Geometry check sheet. Reference: the model listing, model coordinates, mm. Face numbers are marked on the shaded views. Coordinates: 2 decimals unless noted, no trailing zeros. Write each loop counter-clockwise with the first axis right and the second up, starting at its lowest first coordinate (ties: lowest second). Pieces come first, ordered by that corner, then holes. Notation, with made-up numbers: M 42.25,62.25 L 71.25,62.25 A19 cw 71.25,78.25 Z; hole C 53.25,52 d9. An arc over 180 degrees is marked long. Answer as a JSON object with one key per item and string values. Group by question number.
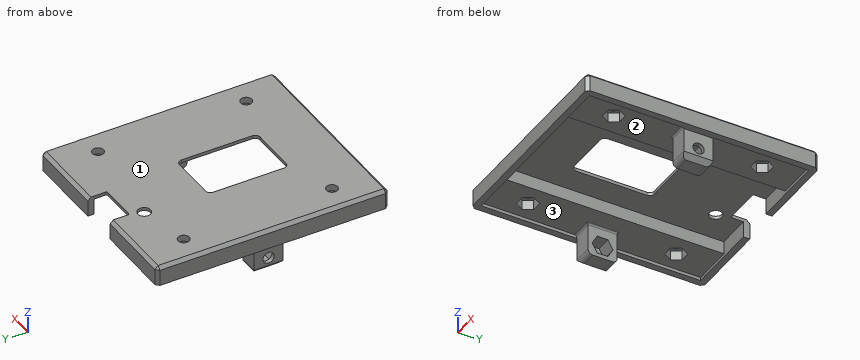
```python
from build123d import *

# Parameters (mm, degrees)
CYLINDER021_R            = 2
CYLINDER021_DEPTH        = 15
BOX014_W                 = 4
BOX014_H                 = 9
BOX014_DEPTH             = 3
PRISM010_DEPTH           = 10
PRISM010_ROLL_ANGLE      = -90.000052
PRISM010_PITCH_ANGLE     = -59.999967
PRISM010_PLACEMENT_ANGLE = 90.000052
CYLINDER019_R            = 1.75
CYLINDER019_DEPTH        = 68
CYLINDER019_PITCH_ANGLE  = 90
BOX013_W                 = 6
BOX013_H                 = 9
BOX013_DEPTH             = 11
CHAMFER008_SIZE          = 1.5
FILLET009_R              = 1.5
BOX012_W                 = 12
BOX012_H                 = 16
BOX012_DEPTH             = 10
PAD021_DEPTH             = 35
CYLINDER005_R            = 1.75
CYLINDER005_DEPTH        = 50
CYLINDER007_R            = 1.75
CYLINDER007_DEPTH        = 50
CYLINDER006_R            = 1.75
CYLINDER006_DEPTH        = 50
CYLINDER004_R            = 1.75
CYLINDER004_DEPTH        = 50
PRISM004_DEPTH           = 10
PRISM005_DEPTH           = 10
PRISM006_DEPTH           = 10
PRISM007_DEPTH           = 10
SKETCH001_W              = 58
SKETCH001_H              = 68
PAD001_DEPTH             = 2
SKETCH002_W              = 33
SKETCH002_H              = 68
PAD002_DEPTH             = 6
BOX009_W                 = 62
BOX009_H                 = 72
BOX009_DEPTH             = 6
CHAMFER001_SIZE          = 1
FILLET010_R              = 0.5


with BuildPart() as cilindro017:
    # Cylinder021 → Cylinder021 (new body)
    with BuildSketch(Plane(origin=(-7, 26, 17), x_dir=(1, 0, 0), z_dir=(0, 0, 1))):
        Circle(CYLINDER021_R)
    extrude(amount=CYLINDER021_DEPTH)


with BuildPart() as cubo014:
    # Box014 → Box014 (new body)
    with BuildSketch(Plane(origin=(-29.75, -4.5, 23), x_dir=(1, 0, 0), z_dir=(0, 0, 1))):
        with Locations((2, 4.5)):
            Rectangle(BOX014_W, BOX014_H)
    extrude(amount=BOX014_DEPTH)


with BuildPart() as prisma010:
    # Prism010 → Prism010 (new body)
    with BuildSketch(Plane.XY):
        Polygon((3.25, 0), (1.625, 2.814583), (-1.625, 2.814583), (-3.25, 0), (-1.625, -2.814583), (1.625, -2.814583), align=None)
    extrude(amount=PRISM010_DEPTH)


with BuildPart() as prisma010_1:
    # Prism010 roll: moved
    add(prisma010.part.rotate(Axis((0, 0, 0), (1, 0, 0)), PRISM010_ROLL_ANGLE))


with BuildPart() as prisma010_2:
    # Prism010 pitch: moved
    add(prisma010_1.part.rotate(Axis((0, 0, 0), (0, 1, 0)), PRISM010_PITCH_ANGLE))


with BuildPart() as prisma010_3:
    # Prism010 placement: moved
    add(prisma010_2.part.moved(Location((-17.5, 0, 18))).rotate(Axis((-17.5, 0, 18), (0, 0, 1)), PRISM010_PLACEMENT_ANGLE))


with BuildPart() as cilindro016:
    # Cylinder019 → Cylinder019 (new body)
    with BuildSketch(Plane.XY):
        Circle(CYLINDER019_R)
    extrude(amount=CYLINDER019_DEPTH)


with BuildPart() as cilindro016_1:
    # Cylinder019 pitch: moved
    add(cilindro016.part.rotate(Axis((0, 0, 0), (0, 1, 0)), CYLINDER019_PITCH_ANGLE))


with BuildPart() as cilindro016_2:
    # Cylinder019 placement: moved
    add(cilindro016_1.part.moved(Location((-34, 0, 18))))


with BuildPart() as fusion016:
    # Box013 → Box013 (new body)
    with BuildSketch(Plane(origin=(-28.75, -4.5, 14), x_dir=(1, 0, 0), z_dir=(0, 0, 1))):
        with Locations((3, 4.5)):
            Rectangle(BOX013_W, BOX013_H)
    extrude(amount=BOX013_DEPTH)

    # Cut028: cut Cilindro016
    add(cilindro016_2.part, mode=Mode.SUBTRACT)

    # Chamfer008
    chamfer008_edges = [fusion016.edges().sort_by_distance(p)[0] for p in [
        (-28.75, 0, 14),
    ]]
    chamfer(chamfer008_edges, length=CHAMFER008_SIZE)

    # Fillet009
    fillet009_edges = [fusion016.edges().sort_by_distance(p)[0] for p in [
        (-25, -4.5, 14),
        (-25, 4.5, 14),
    ]]
    fillet(fillet009_edges, radius=FILLET009_R)

    # Cut029: cut Prisma010
    add(prisma010_3.part, mode=Mode.SUBTRACT)

    # Fusion016: union Cubo014
    add(cubo014.part)


with BuildPart() as part_mirroring032:
    # Part__Mirroring032: instance of Fusion016
    add(fusion016.part.mirror(Plane(origin=(0, 0, 0), x_dir=(0, -1, 0), z_dir=(1, 0, 0))))


with BuildPart() as fusion017:
    # Fusion017 base: copy of Fusion016
    add(fusion016.part)

    # Fusion017: union Part__Mirroring032
    add(part_mirroring032.part)


with BuildPart() as cubo012:
    # Box012 → Box012 (new body)
    with BuildSketch(Plane(origin=(-6, 30, 22), x_dir=(1, 0, 0), z_dir=(0, 0, 1))):
        with Locations((6, 8)):
            Rectangle(BOX012_W, BOX012_H)
    extrude(amount=BOX012_DEPTH)


with BuildPart() as pad021:
    # Sketch018 → Pad021 (new body)
    with BuildSketch(Plane.XY.offset(40)):
        with BuildLine():
            Line((-7, 7), (7, 7))
            ThreePointArc((8.5, 5.5), (8.06066, 6.56066), (7, 7))
            Line((8.5, 5.5), (8.5, -16.5))
            ThreePointArc((7, -18), (8.06066, -17.56066), (8.5, -16.5))
            Line((7, -18), (-7, -18))
            ThreePointArc((-8.5, -16.5), (-8.06066, -17.56066), (-7, -18))
            Line((-8.5, -16.5), (-8.5, 5.5))
            ThreePointArc((-7, 7), (-8.06066, 6.56066), (-8.5, 5.5))
        make_face()
    extrude(amount=-PAD021_DEPTH)


with BuildPart() as cilindro005:
    # Cylinder005 → Cylinder005 (new body)
    with BuildSketch(Plane(origin=(23, 23, -15), x_dir=(1, 0, 0), z_dir=(0, 0, 1))):
        Circle(CYLINDER005_R)
    extrude(amount=CYLINDER005_DEPTH)


with BuildPart() as cilindro007:
    # Cylinder007 → Cylinder007 (new body)
    with BuildSketch(Plane(origin=(23, -23, -15), x_dir=(1, 0, 0), z_dir=(0, 0, 1))):
        Circle(CYLINDER007_R)
    extrude(amount=CYLINDER007_DEPTH)


with BuildPart() as cilindro006:
    # Cylinder006 → Cylinder006 (new body)
    with BuildSketch(Plane(origin=(-23, -23, -15), x_dir=(1, 0, 0), z_dir=(0, 0, 1))):
        Circle(CYLINDER006_R)
    extrude(amount=CYLINDER006_DEPTH)


with BuildPart() as fusion002:
    # Cylinder004 → Cylinder004 (new body)
    with BuildSketch(Plane(origin=(-23, 23, -15), x_dir=(1, 0, 0), z_dir=(0, 0, 1))):
        Circle(CYLINDER004_R)
    extrude(amount=CYLINDER004_DEPTH)

    # Fusion002: union Cilindro005, Cilindro007, Cilindro006
    add(cilindro005.part)
    add(cilindro007.part)
    add(cilindro006.part)


with BuildPart() as prisma004:
    # Prism004 → Prism004 (new body)
    with BuildSketch(Plane(origin=(-23, 23, 0), x_dir=(1, 0, 0), z_dir=(0, 0, 1))):
        Polygon((3.1, 0), (1.55, 2.684679), (-1.55, 2.684679), (-3.1, 0), (-1.55, -2.684679), (1.55, -2.684679), align=None)
    extrude(amount=PRISM004_DEPTH)


with BuildPart() as prisma005:
    # Prism005 → Prism005 (new body)
    with BuildSketch(Plane(origin=(23, 23, 0), x_dir=(1, 0, 0), z_dir=(0, 0, 1))):
        Polygon((3.1, 0), (1.55, 2.684679), (-1.55, 2.684679), (-3.1, 0), (-1.55, -2.684679), (1.55, -2.684679), align=None)
    extrude(amount=PRISM005_DEPTH)


with BuildPart() as prisma006:
    # Prism006 → Prism006 (new body)
    with BuildSketch(Plane(origin=(-23, -23, 0), x_dir=(1, 0, 0), z_dir=(0, 0, 1))):
        Polygon((3.1, 0), (1.55, 2.684679), (-1.55, 2.684679), (-3.1, 0), (-1.55, -2.684679), (1.55, -2.684679), align=None)
    extrude(amount=PRISM006_DEPTH)


with BuildPart() as fusion004:
    # Prism007 → Prism007 (new body)
    with BuildSketch(Plane(origin=(23, -23, 0), x_dir=(1, 0, 0), z_dir=(0, 0, 1))):
        Polygon((3.1, 0), (1.55, 2.684679), (-1.55, 2.684679), (-3.1, 0), (-1.55, -2.684679), (1.55, -2.684679), align=None)
    extrude(amount=PRISM007_DEPTH)

    # Fusion004: union Prisma004, Prisma005, Prisma006
    add(prisma004.part)
    add(prisma005.part)
    add(prisma006.part)


with BuildPart() as fusion004_1:
    # Fusion004 placement: moved
    add(fusion004.part.moved(Location((0, 0, 17))))


with BuildPart() as pad001:
    # Sketch001 → Pad001 (new body)
    with BuildSketch(Plane(origin=(0, 0, 23), x_dir=(1, 0, 0), z_dir=(0, 0, -1))):
        Rectangle(SKETCH001_W, SKETCH001_H)
    extrude(amount=-PAD001_DEPTH)


with BuildPart() as fusion003:
    # Sketch002 → Pad002 (new body)
    with BuildSketch(Plane(origin=(0, 0, 23), x_dir=(1, 0, 0), z_dir=(0, 0, -1))):
        Rectangle(SKETCH002_W, SKETCH002_H)
    extrude(amount=-PAD002_DEPTH)

    # Fusion003: union Pad001
    add(pad001.part)


with BuildPart() as fusion003_1:
    # Fusion003 placement: moved
    add(fusion003.part.moved(Location((0, 0, -1))))


with BuildPart() as obj1:
    # Box009 → Box009 (new body)
    with BuildSketch(Plane(origin=(-31, -36, 23), x_dir=(1, 0, 0), z_dir=(0, 0, 1))):
        with Locations((31, 36)):
            Rectangle(BOX009_W, BOX009_H)
    extrude(amount=BOX009_DEPTH)

    # Chamfer001
    chamfer001_edges = [obj1.edges().sort_by_distance(p)[0] for p in [
        (-31, -36, 26),
        (-31, 0, 29),
        (-31, 36, 26),
        (31, -36, 26),
        (31, 0, 29),
        (31, 36, 26),
        (0, -36, 29),
        (0, 36, 29),
    ]]
    chamfer(chamfer001_edges, length=CHAMFER001_SIZE)

    # Cut004: cut Fusion003
    add(fusion003_1.part, mode=Mode.SUBTRACT)

    # Cut005: cut Fusion004
    add(fusion004_1.part, mode=Mode.SUBTRACT)

    # Cut006: cut Fusion002
    add(fusion002.part, mode=Mode.SUBTRACT)

    # Cut023: cut Pad021
    add(pad021.part, mode=Mode.SUBTRACT)

    # Cut027: cut Cubo012
    add(cubo012.part, mode=Mode.SUBTRACT)

    # Fusion018: union Fusion017
    add(fusion017.part)

    # Fillet010
    fillet010_edges = [obj1.edges().sort_by_distance(p)[0] for p in [
        (-6, 30, 28.5),
        (6, 30, 28.5),
        (-24.25, 4.5, 24),
        (-22.75, 0, 24),
        (-24.25, -4.5, 24),
        (28.875, -4.5, 24),
        (24.25, -4.5, 24),
        (22.75, 0, 24),
        (24.25, 4.5, 24),
    ]]
    fillet(fillet010_edges, radius=FILLET010_R)

    # Cut032: cut Cilindro017
    add(cilindro017.part, mode=Mode.SUBTRACT)


solid = obj1.part
```
1) Section check A-A (x = -18.5). Record the cut outline in (y, z).
2) Section check B-B (y = 10.5). Record the cut outline in (x, z), then the cut area to 3 significant figures.
3) Section check C-C (y = 0). State how many separate pieces and enclosed holes the cut face has, then the cut area to 3 significant figures.
4) Go/stop test with flat-tipped pins: pin 1 Ø12 at (x, y) = (7.5, 1.5) entering from -Z; pin 2 Ø0.5 at (x, z) = (0.5, 28.5) entering from +Y; pin 3 Ø5 at (x, z) = (26.5, 17.5) entering from +Y. Record where each tip stops, or that it passes through.
5) Draft check along X on the marked faces 1, 2 and 3. Enter one of: +X half, -X half, draft (parallel to the pull), parting line (faces both ways), or undercut.
6) Material ranges on probe 1 along X at (y, z) = (23, 27.6); probe 2 along Y at (x, z) = (-7, 26.25); probe 3 along X at (y, z) = (23, 28.1), recorded low to high. Write a range as [from, to].
Entries:
{
 "1": {"outline": "M -36,23 L -34,23 L -34,24 L 34,24 L 34,23 L 36,23 L 36,28 L 35,29 L -35,29 L -36,28 Z"},
 "2": {"outline": "M -31,23 L -29,23 L -29,24 L -16.5,24 L -16.5,28 L 16.5,28 L 16.5,24 L 29,24 L 29,23 L 31,23 L 31,28 L 30,29 L -30,29 L -31,28 Z", "area": "181 mm^2"},
 "3": {"separate pieces": "4", "enclosed holes": "0", "area": "220 mm^2"},
 "4": {"pin 1": "z = 28", "pin 2": "y = 30", "pin 3": "y = 4.5"},
 "5": {"face 1": "draft", "face 2": "undercut", "face 3": "undercut"},
 "6": {"probe 1": "[-31, -24.75], [-21.25, -16.5], [16.5, 21.25], [24.75, 31]", "probe 2": "[-36, -34], [34, 36]", "probe 3": "[-30.9, -24.75], [-21.25, 21.25], [24.75, 30.9]"}
}
